Check sheet for the modelled part. Datum: model origin and axes. Units: mm. Face numbers are marked on the shaded views. Round coordinates to 2 decimals unless told otherwise and drop trailing zeros. Write each loop counter-clockwise with the first axis right and the second up, starting at its lowest first coordinate (ties: lowest second). Pieces come first, ordered by that corner, then holes. Notation, with made-up numbers: M -14.5,-39.5 L 29.5,-39.5 A9 ccw 29.5,-35.5 Z; hole C -3.75,-3 d4. An arc over 180 degrees is marked long. Answer in a Markdown table with one row per item.
```python
from build123d import *

# Parameters (mm, degrees)
F3_DEPTH = 65.786
F4_SIZE  = 2.53999


# Not quite as in the source:
# - a fillet or chamfer is up to 0.001 mm smaller than in the source, because OpenCascade refuses the exact size


with BuildPart() as f1:
    # F0 (on Front) → F1 (revolve)
    with BuildSketch(Plane.XZ):
        with BuildLine():
            Line((-39.4843606797, -37.7460680902), (-31.8643606797, -37.7460680902))
            Line((-31.8643606797, -37.7460680902), (-31.8643606797, -19.9660680902))
            Line((-31.8643606797, -19.9660680902), (-0.1143606797, -19.9660680902))
            Line((-0.1143606797, -19.9660680902), (-0.1143606797, -14.8860680902))
            Line((-0.1143606797, -14.8860680902), (-35.6743606797, -14.8860680902))
            Line((-35.6743606797, -14.8860680902), (-35.6743606797, -9.8060680902))
            Line((-35.6743606797, -9.8060680902), (-39.4843606797, -9.8060680902))
            ThreePointArc((-39.4843606797, -9.8060680902), (-37.8052347612, -23.7760680902), (-39.4843606797, -37.7460680902))
        make_face()
    revolve(axis=Axis((-0.1143606797, 0, -17.4260680902), (0, 0, -1)))

    # F2 (on Top) → F3 (cut)
    with BuildSketch(Plane.XY):
        with BuildLine():
            add(Edge.make_bspline(
                [(10.16, -23.495), (10.16, -15.7960341604), (-5.08, -19.6455170802), (-20.32, -23.495), (-5.08, -27.3444829198), (10.16, -31.1939658396), (10.16, -23.495)],
                knots=[0, 0, 0, 2.0943951024, 2.0943951024, 4.1887902048, 4.1887902048, 6.2831853072, 6.2831853072, 6.2831853072], degree=2, weights=[1, 0.5, 1, 0.5, 1, 0.5, 1]))
        make_face()
    extrude(amount=-F3_DEPTH, mode=Mode.SUBTRACT)

    # F4 (size 2.54 in the source; OpenCascade refuses exactly that, so slightly less here)
    f4_edges = [f1.edges().sort_by_distance(p)[0] for p in [
        (35.445639, 0, -14.886068),
        (35.445639, 0, -9.806068),
        (-35.674361, 0, -12.346068),
    ]]
    chamfer(f4_edges, length=F4_SIZE)


solid = f1.part
```
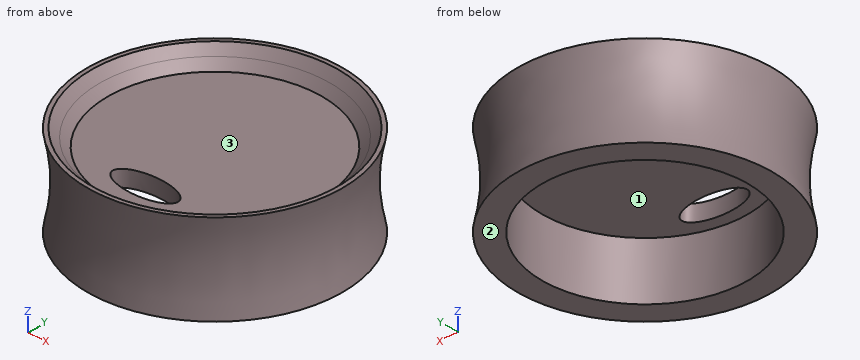
1. Section check B-B, the plane z = -23.25. Record the cut outline in (x, y), and give its area (3 significant figures).
Found:
| item | result |
|---|---|
| outline | C -0.11,0 d75.39; hole C -0.11,0 d63.5 |
| area | 1,300 mm2 |
2. Draft check along Y on the marked faces 1, 2 and 3. Enter one of: +Y half, -Y half, draft (parallel to the pull), parting line (faces both ways), or undercut.
Found:
| item | result |
|---|---|
| face 1 | undercut |
| face 2 | draft |
| face 3 | undercut |
3. Scan lines: L1, parallel to Z at x = -12, y = 17.5; L2, parallel to X at y = 9, z = -35.25; L3, parallel to X at y = 21, z = -34.75. Record each from-to range of solid material in increasing order.
Found:
| item | result |
|---|---|
| L1 | z = -19.97 to -14.89 |
| L2 | x = -37.87 to -30.56, 30.33 to 37.65 |
| L3 | x = -32.65 to -23.93, 23.7 to 32.42 |
4. Go/stop test with flat-tipped pins: pin 1 (2 mm diameter, centred on x = -4.5, z = -27, fed in from -Y); pin 2 (8 mm diameter, centred on x = 11, y = 24.5, fed in from +Z); pin 3 (8 mm diameter, centred on y = 25.5, z = -33.5, fed in from -X). Record where each tip stops, or that it passes through.
Found:
| item | result |
|---|---|
| pin 1 | stops at y = -37.64 |
| pin 2 | stops at z = -14.89 |
| pin 3 | stops at x = -32.18 |
